For this review, take the finished solid that the model builds, in its own axes (mm). A direction names the side the tool comes from. Round coordinates to 2 decimals unless told otherwise and drop trailing zeros. Order: outer loops, then holes, each group sorted by start corner. A loop starts at its lowest first (then second) coordinate and runs counter-clockwise, first axis right, second up. Notation, with made-up numbers: M 72,12 L 85,12 A24 ccw 85,41 Z; hole C 6.5,-30 d1. An arc over 180 degrees is marked long. Use a Markdown table: item, result.
Autodesk Inventor part; units mm, degrees
ref_plane "YZ Plane" through (0, 0, 0) normal (1, 0, 0) x (0, 1, 0)
ref_plane "XZ Plane" through (0, 0, 0) normal (0, 1, 0) x (-1, 0, 0)
ref_plane "XY Plane" through (0, 0, 0) normal (0, 0, 1) x (1, 0, 0)
sketch "Sketch1" plane through (0, 0, 0) normal (0, 0, 1) x (1, 0, 0)
  line L0 (-50, -100) -> (50, -100)
  line L1 (50, -100) -> (50, 100)
  line L2 (50, 100) -> (-50, 100)
  line L3 (-50, 100) -> (-50, -100)
  line L4 (-50, -100) -> (50, 100) construction
  line L5 (50, -100) -> (-50, 100) construction
  point P0 (0, 0)
  dimension "d0" = 100
  dimension "d1" = 200
extrude "Extrusion1" add sketch "Sketch1" along normal blind 5
sketch "Sketch2" plane through (-50, 100, 0) normal (0, 1, 0) x (1, 0, 0)
  line L0 (0, 0) -> (100, 0)
  line L1 (0, 0) -> (49.9986, 49.9986)
  line L2 (49.9986, 49.9986) -> (53.5341, 46.463)
  line L3 (53.5341, 46.463) -> (3.5355, -3.5355)
  line L4 (3.5355, -3.5355) -> (0, 0)
  line L5 (0, 0) -> (70.7086, 0) construction
  line L6 (100.108, -0.1109) -> (53.5341, 46.463)
  line L7 (53.5341, 46.463) -> (49.9986, 42.9275)
  line L8 (49.9986, 42.9275) -> (96.5724, -3.6464)
  line L9 (96.5724, -3.6464) -> (100.108, -0.1109)
  point P0 (50, 0)
  point P1 (49.9986, 42.9275)
  dimension "d4" = 45
  dimension "d5" = 5
  dimension "d6" = 5
extrude "Extrusion2" add sketch "Sketch2" against normal blind 30 contours L1 L2 L3 L0 | L0 L3 L4 | L8 L3 L6 L0 | L0 L6 L9 L8
sketch "Sketch6" plane through (0, 0, 5) normal (0, 0, 1) x (1, 0, 0)
  line L0 (4.9986, 75) -> (-5.0014, 75)
  line L1 (-25.0014, 55) -> (-25.0014, 45)
  line L2 (-5.0014, 25) -> (4.9986, 25)
  line L3 (24.9986, 45) -> (24.9986, 55)
  line L4 (24.9986, 75) -> (-25.0014, 25) construction
  line L5 (-25.0014, 75) -> (24.9986, 25) construction
  arc A0 (4.9986, 25) -> (24.9986, 45) centre (4.9986, 45) ccw
  arc A1 (24.9986, 55) -> (4.9986, 75) centre (4.9986, 55) ccw
  arc A2 (-5.0014, 75) -> (-25.0014, 55) centre (-5.0014, 55) ccw
  arc A3 (-25.0014, 45) -> (-5.0014, 25) centre (-5.0014, 45) ccw
  point P0 (0, 0)
  point P1 (-0.0014, 50)
  dimension "d21" = 50
  dimension "d22" = 50
  dimension "d23" = 20
extrude "Extrusion6" cut sketch "Sketch6" against normal blind 5
sketch "Sketch10" plane through (-50, 100, 5) normal (0, 1, 0) x (1, 0, 0)
  line L0 (0, 5) -> (7.0711, 5)
  line L1 (49.9986, 54.9986) -> (99.9971, 5)
  line L2 (0, 5) -> (49.9986, 54.9986)
  line L3 (49.9986, 54.9986) -> (46.463, 58.5341)
  line L4 (46.463, 58.5341) -> (-3.5355, 8.5355)
  line L5 (-3.5355, 8.5355) -> (0, 5)
  line L6 (100, 4.7812) -> (100, 0)
  line L7 (100, 4.7812) -> (49.9986, 54.9986)
  line L8 (49.9986, 54.9986) -> (53.5417, 58.5265)
  line L9 (53.5417, 58.5265) -> (103.5431, 8.3091)
  line L10 (103.5431, 8.3091) -> (100, 4.7812)
  line L11 (92.926, 5) -> (49.9986, 47.9275)
  line L12 (100, 0) -> (0, 0)
  line L13 (0, 0) -> (100, 0)
  point P0 (50, 5)
  dimension "d33" = 5
  dimension "d34" = 5
extrude "Extrusion9" add sketch "Sketch10" against normal blind 3
sketch "Sketch12" plane through (-50, 100, 5) normal (0, 1, 0) x (1, 0, 0)
  circle A0 centre (89.5, 8) radius 4.5
  circle A1 centre (10.5, 8) radius 4.5
  line L0 (49.9986, 47.9275) -> (7.0711, 5)
  circle A2 centre (49.9986, 47.9275) radius 4.5
  point P0 (50, 5)
  dimension "d38" = 9
  dimension "d39" = 9
  dimension "d41" = 9
extrude "Extrusion10" add sketch "Sketch12" along normal blind 14
properties part number "fixation_v09"
Q1. Clearance check with flat-ended pins moving along their axes: pin 1 (5.5 mm diameter, centred on x = 1.5, z = 2.5, fed in from +Y); pin 2 (4 mm diameter, centred on y = 46.5, z = 1.5, fed in from -X); pin 3 (2 mm diameter, centred on x = -27.5, y = -12.5, fed in from -Z); pin 4 (5 mm diameter, centred on x = -23, z = -40.5, fed in from -Y). State where each tip first meets the part, or that it passes through.
Determined:
| item | result |
|---|---|
| pin 1 | stops at y = 100 |
| pin 2 | stops at x = -50 |
| pin 3 | stops at z = 0 |
| pin 4 | passes through |
Q2. Draft analysis for pull direction Z (two halves, no side actions). For faces 6 (the flat face through (38, 100, -3)), 7 (the flat face through (-27, 97, -27)), 8 (the flat face through (-25, 84, -25)), state which applies: pulls with the +Z half, pulls with the -Z half, needs draft (parallel to the pull), parting line crosses it, or undercut.
Determined:
| item | result |
|---|---|
| face 6 | undercut |
| face 7 | needs draft |
| face 8 | pulls with the -Z half |
Q3. Add section A-A (y = 39.5). Write out the cut boundary in (x, z).
Determined:
| item | result |
|---|---|
| outline | M -50,0 L -24.23,0 L -24.23,5 L -50,5 Z; M 24.23,0 L 50,0 L 50,5 L 24.23,5 Z |
Q4. Wall thickness on line 1 along Y through (x, z) = (30, -18.5); line 2 along Z through (x, y) = (-7.5, -20); line 3 along Z through (x, y) = (-22, 94.5): over which ranges is each line inside the solid? List them lowest first. Write a range as [from, to].
Determined:
| item | result |
|---|---|
| line 1 | y = [70, 100] |
| line 2 | z = [0, 5] |
| line 3 | z = [-28, -20.93], [0, 5] |
Q5. Machinability: for faces 1 (the flat face through (0, 100, -40)), 2 (the cylindrical face through (-18.987, 69.297, 2.535)), 3 (the cylindrical face through (18.98, 30.7, 2.54)), 4 (the cylindrical face through (43.792, 106.902, -1.648)), 5 (the flat face through (-11, 70, -33)), which of the approach directions +Z, -Z, +X, -X, +Y, -Y give a long, thin tool a straight path to every point of the face, cutting with its end or side? Answer none if there is none.
Determined:
| item | result |
|---|---|
| face 1 | -Y |
| face 2 | +Z |
| face 3 | +Z, -Z |
| face 4 | +Y |
| face 5 | -Z, +X, -X, -Y |
Q6. Add section D-D (z = -22.5). Write out the cut boundary in (x, y).
Determined:
| item | result |
|---|---|
| outline | M -34.57,97 L -27.5,97 L -27.5,70 L -20.43,70 L -20.43,100 L -34.57,100 Z; M 20.43,70 L 27.5,70 L 27.5,97 L 34.43,97 L 34.43,100 L 20.43,100 Z |
Q7. Add section B-B (x = 17.5). Write out the cut boundary in (y, z).
Determined:
| item | result |
|---|---|
| outline | M -100,0 L 29.39,0 L 29.39,5 L -100,5 Z; M 70,-32.5 L 97,-32.5 L 97,-39.51 L 100,-39.51 L 100,-25.43 L 70,-25.43 Z; M 70.61,0 L 100,0 L 100,5 L 70.61,5 Z |
